For this review, use the dimensioned drawing (mm, ordinates from the lowest corner) and the shaded views. A direction names the side the tool comes from. Coordinates: 2 decimals unless noted, no trailing zeros. Order: outer loops, then holes, each group sorted by start corner. A loop starts at its lowest first (then second) coordinate and runs counter-clockwise, first axis right, second up. Notation, with made-up numbers: M 76,-27 L 106,-27 A22 cw 106,6 Z; hole C 31,75.5 d1. An arc over 180 degrees is marked long. Write each question's results on one line, items separated by ' | '.
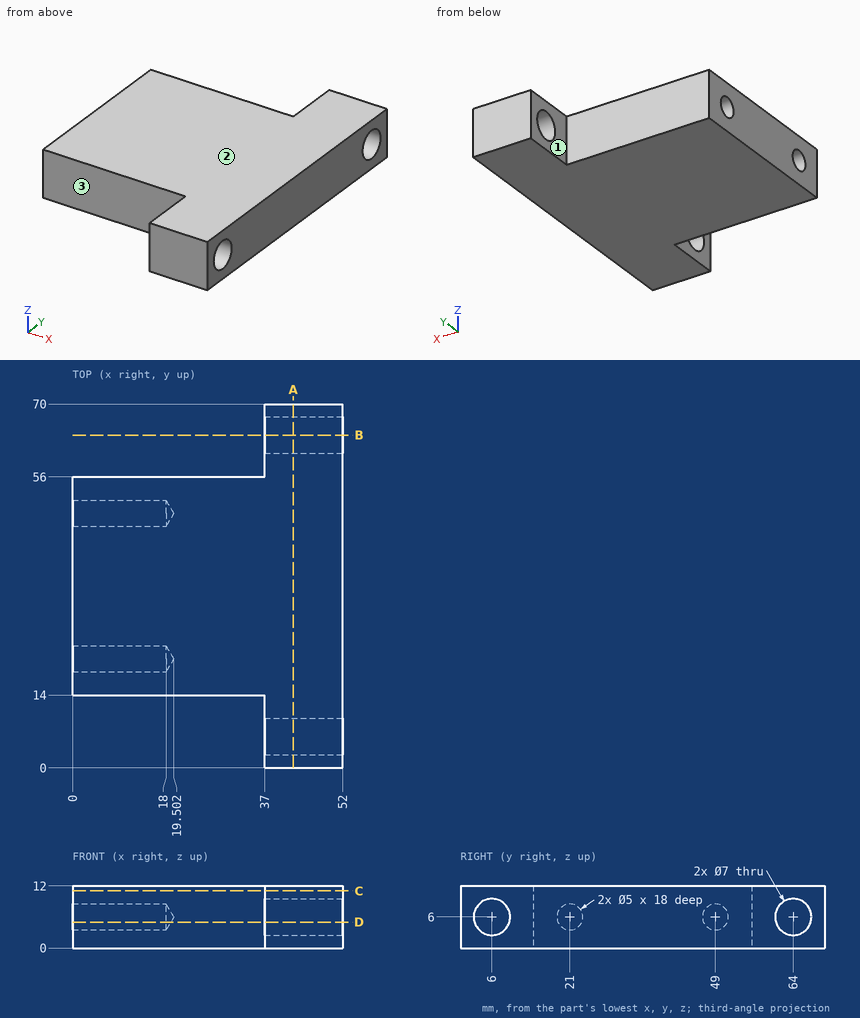
1) For pin 1 (1 mm diameter, centred on y = 40, z = 10.5, fed in from -X); pin 2 (1 mm diameter, centred on x = 10, z = 4, fed in from -Y); pin 3 (3.5 mm diameter, centred on y = 61, z = 7.5, fed in from -X); pin 4 (6 mm diameter, centred on x = 26, z = 5.5, fed in from +Y), all flat-tipped, find the tip position at first contact; note any pin that passes through.
Solutions:
pin 1: x = 0 | pin 2: y = 14 | pin 3: x = 37 | pin 4: y = 56
2) Take a section at C-C on z = 11. State the section outline as (x, y) points, plus the area to 3 significant figures.
Solutions:
outline: M 0,14 L 37,14 L 37,0 L 52,0 L 52,70 L 37,70 L 37,56 L 0,56 Z | area: 2,600 mm2
3) Take a section at B-B on y = 64. State the section outline as (x, z) points, plus the area to 3 significant figures.
Solutions:
outline: M 37,0 L 52,0 L 52,2.5 L 37,2.5 Z; M 37,9.5 L 52,9.5 L 52,12 L 37,12 Z | area: 75.0 mm2
4) Take a section at D-D on z = 5. Count the separate pieces of the cut face and the enclosed holes in it, plus the area to 3 significant figures.
Solutions:
separate pieces: 3 | enclosed holes: 0 | area: 2,230 mm2
5) For the marked faces 1, 2 and 3, list the 3-axis set-ups (+Z, -Z, +X, -X, +Y, -Y) from which the entire face can be reached by the end or side of a thin tool; tool diameter is ignored.
Solutions:
face 1: +Z, -Z, -X, +Y | face 2: +Z, +X, -X, +Y, -Y | face 3: +Z, -Z, -X, -Y
6) To check wall thickness, follow line 1 along Y through (x, z) = (45.5, 6); line 2 along Y through (x, z) = (4.5, 6); line 3 along Y through (x, z) = (2, 2). State the ranges of each line that lie inside material, in increasing order.
Solutions:
line 1: 0 to 2.5, 9.5 to 60.5, 67.5 to 70 | line 2: 14 to 18.5, 23.5 to 46.5, 51.5 to 56 | line 3: 14 to 56
7) Take a section at A-A on x = 42.5. State the section outline as (y, z) points, plus the area to 3 significant figures.
Solutions:
outline: M 0,0 L 70,0 L 70,12 L 0,12 Z; hole C 6,6 d7; hole C 64,6 d7 | area: 763 mm2
